Check sheet for the modelled part. Datum: model origin and axes. Units: mm. A direction names the side the tool comes from. Coordinates: 2 decimals unless noted, no trailing zeros. Loops run counter-clockwise (first coordinate to the right, second up) from the corner with the lowest first, then second, coordinate; pieces in that order, holes last. Notation, with made-up numbers: (84, 69) -> (117, 69) arc R17 cw to (117, 76) -> close; hole circle Ø2 at (2.5, 30). An arc over 180 degrees is marked (long way). Use one line per item in the form item = value.
from build123d import *

# Parameters (mm, degrees)
F1_W     = 24
F1_H     = 11
F2_DEPTH = 5


with BuildPart() as f2:
    # F1 (on face) → F2 (new body)
    with BuildSketch(Plane.XZ):
        Polygon((-4.942675, 15.304768), (-4.942675, 22.984039), (19.057325, 22.984039), (19.057325, 11.984039), (17.873291, 11.984039), (17.873291, 6.802615), (19.057325, 6.802615), (19.057325, -3.695232), (30.870639, -3.695232), (30.870639, -0.695232), (35.870639, -0.695232), (35.870639, 43.304768), (30.870639, 43.304768), (30.870639, 46.304768), (-19.129361, 46.304768), (-19.129361, 43.304768), (-24.129361, 43.304768), (-24.129361, -0.695232), (-19.129361, -0.695232), (-19.129361, -3.695232), (-4.942675, -3.695232), (-4.942675, 4.304768), (-6.126709, 4.304768), (-6.126709, 15.304768), align=None)
        with Locations((5.873291, 32.804768)):
            Rectangle(F1_W, F1_H, mode=Mode.SUBTRACT)
    extrude(amount=F2_DEPTH)


solid = f2.part
(1) Section check C-C, the plane y = -3.6. Record the boundary of the cut face in (x, z).
Established:
outline = (-24.13, -0.7) -> (-19.13, -0.7) -> (-19.13, -3.7) -> (-4.94, -3.7) -> (-4.94, 4.3) -> (-6.13, 4.3) -> (-6.13, 15.3) -> (-4.94, 15.3) -> (-4.94, 22.98) -> (19.06, 22.98) -> (19.06, 11.98) -> (17.87, 11.98) -> (17.87, 6.8) -> (19.06, 6.8) -> (19.06, -3.7) -> (30.87, -3.7) -> (30.87, -0.7) -> (35.87, -0.7) -> (35.87, 43.3) -> (30.87, 43.3) -> (30.87, 46.3) -> (-19.13, 46.3) -> (-19.13, 43.3) -> (-24.13, 43.3) -> close; hole (-6.13, 27.3) -> (17.87, 27.3) -> (17.87, 38.3) -> (-6.13, 38.3) -> close
(2) Scan lines: line 1 along X through (y, z) = (-3.65, 3); line 2 along X through (y, z) = (-1.05, 7.5); line 3 along Z through (x, y) = (17.5, -1.1). Record each from-to range of solid material in increasing order.
Established:
line_1 = -24.13 to -4.94, 19.06 to 35.87
line_2 = -24.13 to -6.13, 17.87 to 35.87
line_3 = 22.98 to 27.3, 38.3 to 46.3
(3) Section check B-B, the plane z = 3. Record the boundary of the cut face in (x, y).
Established:
outline = (-24.13, -5) -> (-4.94, -5) -> (-4.94, 0) -> (-24.13, 0) -> close; (19.06, -5) -> (35.87, -5) -> (35.87, 0) -> (19.06, 0) -> close
(4) Mould release check, pull along X, two halves, no side actions. Record for faces 1 (the flat face through (5, -5, 27)), 2 (the flat face through (18.5, -2.5, 11.984)), 3 (the flat face through (-4.943, -2, 19)), 4 (the flat face through (30.871, -2, -2)): +X half, -X half, draft (parallel to the pull), parting line (faces both ways), or undercut.
Established:
face_1 = draft
face_2 = undercut
face_3 = undercut
face_4 = +X half
(5) Section check A-A, the plane x = 6. Record the boundary of the cut face in (y, z), plus the area to 3 significant figures.
Established:
outline = (-5, 22.98) -> (0, 22.98) -> (0, 27.3) -> (-5, 27.3) -> close; (-5, 38.3) -> (0, 38.3) -> (0, 46.3) -> (-5, 46.3) -> close
area = 61.6 mm²
(6) Tool access check on faces 5 (the flat face through (33, -2, 43.305)), 6 (the flat face through (18.5, -2.5, 6.803)), 7 (the flat face through (6, -2, 38.305)), 8 (the flat face through (33, -2, -0.695)). Record the directions out of +Z, -Z, +X, -X, +Y, -Y that give a thin tool (end or side, any length) a straight path to the whole face; none if there is none.
Established:
face_5 = +Z, +X, +Y, -Y
face_6 = -Z, +Y, -Y
face_7 = +Y, -Y
face_8 = -Z, +X, +Y, -Y
(7) Go/stop test with flat-tipped pins: P1, Ø1.5, axis at y = -2, z = 44.5, coming from the -X side; P2, Ø0.6, axis at x = 18.5, y = -1.5, coming from the -Z side; P3, Ø1.5, axis at y = -3, z = 45, coming from the +X side. Record where each tip stops, or that it passes through.
Established:
P1 = -19.13
P2 = 6.8
P3 = 30.87
